Read the model definition and answer for the solid it produces. Units are mm, in the model's axes. Give positions to 0.01 mm unless a question says otherwise; leave off trailing zeros. Write each loop counter-clockwise with the first axis right and the second up, starting at its lowest first coordinate (ties: lowest second). Pieces come first, ordered by that corner, then holes. Notation, with made-up numbers: M -18,83.25 L 8,83.25 A26 cw 8,107.25 Z; hole C 76.25,48.5 d3. An arc over 180 degrees is marked long. Use a Markdown table: item, result. Add a question column.
Item 1: Consider probe 1 along Y at (x, z) = (18, 38.5); probe 2 along Z at (x, y) = (-62, 8.25) (3 decimals); probe 3 along Z at (x, y) = (-63.5, 7.75). Determine where each line is inside the solid, lowest interval first. Write a range as [from, to].
Item 2: Given P1, Ø3, axis at x = -23, z = 36, coming from the +Y side; P2, Ø2, axis at x = -19.5, y = 6, coming from the -Z side; P3, Ø5, axis at x = -34, y = 4, coming from the -Z side, each flat-ended and moving along its own axis, determine where each tip first touches the part or whether it passes through.
Item 3: A cutting plane is placed at C-C on z = 34.5. Determine the outline of the cut face in (x, y), then the cut area to 3 significant figures.
Item 4: A cutting plane is placed at B-B on y = 5.25. Determine the outline of the cut face in (x, z).
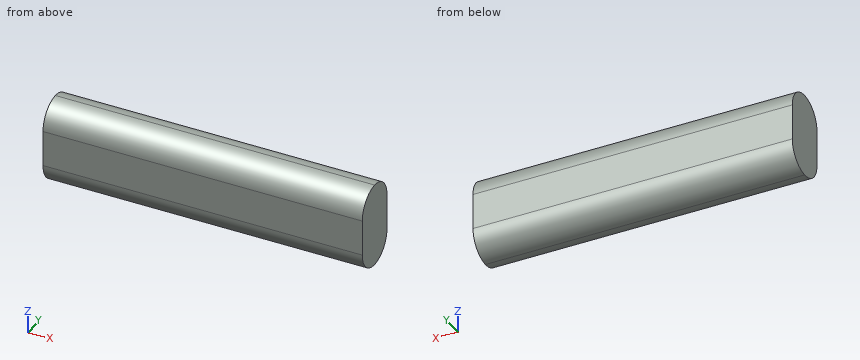
from build123d import *

# Parameters (mm, degrees)
SKETCH2_W           = 132
SKETCH2_H           = 35
BOSS_EXTRUDE1_DEPTH = 20
FILLET1_R           = 10


with BuildPart() as part:
    # Sketch2 → Boss-Extrude1 (new body)
    with BuildSketch(Plane(origin=(0, 0, 0), x_dir=(1, 0, 0), z_dir=(0, 1, 0))):
        with Locations((-21.769456002, -22.770691578)):
            Rectangle(SKETCH2_W, SKETCH2_H)
    extrude(amount=BOSS_EXTRUDE1_DEPTH)

    # Fillet1
    fillet1_edges = [part.edges().sort_by_distance(p)[0] for p in [
        (-21.769456002, 0, 40.270691578),
        (-21.769456002, 0, 5.270691578),
        (-21.769456002, 20, 5.270691578),
        (-21.769456002, 20, 40.270691578),
    ]]
    fillet(fillet1_edges, radius=FILLET1_R - 0.0001)  # a hair under: the kernel refuses the full size


solid = part.part
Filled in:
| question | item | result |
|---|---|---|
| 1 | probe 1 | [4.32, 15.68] |
| 1 | probe 2 | [5.425, 40.116] |
| 1 | probe 3 | [5.53, 40.01] |
| 2 | P1 | y = 19.06 |
| 2 | P2 | z = 5.73 |
| 2 | P3 | z = 5.9 |
| 3 | outline | M -87.77,0.94 L 44.23,0.94 L 44.23,19.06 L -87.77,19.06 Z |
| 3 | area | 2,390 mm² |
| 4 | outline | M -87.77,6.47 L 44.23,6.47 L 44.23,39.07 L -87.77,39.07 Z |
